```python
from build123d import *

# Parameters (mm, degrees)
SKETCH1_W           = 200
SKETCH1_H           = 200
BOSS_EXTRUDE1_DEPTH = 10
SKETCH2_R           = 5
SKETCH2_R_2         = 2.15
CUT_EXTRUDE1_DEPTH  = 142.774468788
SKETCH3_W           = 20
SKETCH3_H           = 5
SKETCH4_R           = 12.5
SKETCH4_R_2         = 5
SKETCH4_R_3         = 7.5
SKETCH4_R_4         = 2.15
CUT_EXTRUDE2_DEPTH  = 5
BOSS_EXTRUDE3_DEPTH = 1


with BuildPart() as part:
    # Sketch1 → Boss-Extrude1 (new body)
    with BuildSketch(Plane.XY):
        Rectangle(SKETCH1_W, SKETCH1_H)
    extrude(amount=BOSS_EXTRUDE1_DEPTH)

    # Sketch2 → Cut-Extrude1 (cut, through all)
    with BuildSketch(Plane.XY.offset(10)):
        with Locations((-40, 30)):
            Circle(SKETCH2_R)
        with Locations((40, 30)):
            Circle(SKETCH2_R)
        with Locations((40, -30)):
            Circle(SKETCH2_R)
        with Locations((-40, -30)):
            Circle(SKETCH2_R)
        with Locations((-30, 40)):
            Circle(SKETCH2_R)
        with Locations((30, 40)):
            Circle(SKETCH2_R)
        with Locations((30, -40)):
            Circle(SKETCH2_R)
        with Locations((-30, -40)):
            Circle(SKETCH2_R)
        with Locations((-56.6, 90.4)):
            Circle(SKETCH2_R_2)
        with Locations((-90.4, 56.6)):
            Circle(SKETCH2_R_2)
        with Locations((-90.4, -56.6)):
            Circle(SKETCH2_R_2)
        with Locations((-56.6, -90.4)):
            Circle(SKETCH2_R_2)
        with Locations((56.6, -90.4)):
            Circle(SKETCH2_R_2)
        with Locations((90.4, -56.6)):
            Circle(SKETCH2_R_2)
        with Locations((90.4, 56.6)):
            Circle(SKETCH2_R_2)
        with Locations((56.6, 90.4)):
            Circle(SKETCH2_R_2)
    extrude(amount=-CUT_EXTRUDE1_DEPTH, mode=Mode.SUBTRACT)

    # Sketch3 → Cut-Revolve1 (revolve, cut)
    with BuildSketch(Plane(origin=(0, 0, 0), x_dir=(1, 0, 0), z_dir=(0, 1, 0))):
        with Locations((0, -4.492265688)):
            Rectangle(SKETCH3_W, SKETCH3_H)
    revolve(axis=Axis((0, 0, 354.492265688), (1, 0, 0)), mode=Mode.SUBTRACT)

    # Sketch4 → Cut-Extrude2 (cut)
    # profile 1 of 30: a face of its own
    with BuildSketch(Plane.XY.offset(10)):
        with Locations((40, 30)):
            Circle(SKETCH4_R)
    # profile 2 of 30: a face of its own
    with BuildSketch(Plane.XY.offset(10)):
        with Locations((30, 40)):
            Circle(SKETCH4_R)
        with Locations((30, 40)):
            Circle(SKETCH4_R_2, mode=Mode.SUBTRACT)
    # profile 3 of 30: a face of its own
    with BuildSketch(Plane.XY.offset(10)):
        with Locations((30, 40)):
            Circle(SKETCH4_R)
        with Locations((30, 40)):
            Circle(SKETCH4_R_2, mode=Mode.SUBTRACT)
    # profile 4 of 30: a face of its own
    with BuildSketch(Plane.XY.offset(10)):
        with Locations((40, 30)):
            Circle(SKETCH4_R)
        with Locations((40, 30)):
            Circle(SKETCH4_R_2, mode=Mode.SUBTRACT)
    # profile 5 of 30: a face of its own
    with BuildSketch(Plane.XY.offset(10)):
        with Locations((30, 40)):
            Circle(SKETCH4_R)
    # profile 6 of 30: a face of its own
    with BuildSketch(Plane.XY.offset(10)):
        with Locations((40, 30)):
            Circle(SKETCH4_R)
        with Locations((40, 30)):
            Circle(SKETCH4_R_2, mode=Mode.SUBTRACT)
    # profile 7 of 30: a face of its own
    with BuildSketch(Plane.XY.offset(10)):
        with Locations((30, -40)):
            Circle(SKETCH4_R)
    # profile 8 of 30: a face of its own
    with BuildSketch(Plane.XY.offset(10)):
        with Locations((40, -30)):
            Circle(SKETCH4_R)
        with Locations((40, -30)):
            Circle(SKETCH4_R_2, mode=Mode.SUBTRACT)
    # profile 9 of 30: a face of its own
    with BuildSketch(Plane.XY.offset(10)):
        with Locations((30, -40)):
            Circle(SKETCH4_R)
        with Locations((30, -40)):
            Circle(SKETCH4_R_2, mode=Mode.SUBTRACT)
    # profile 10 of 30: a face of its own
    with BuildSketch(Plane.XY.offset(10)):
        with Locations((40, -30)):
            Circle(SKETCH4_R)
        with Locations((40, -30)):
            Circle(SKETCH4_R_2, mode=Mode.SUBTRACT)
    # profile 11 of 30: a face of its own
    with BuildSketch(Plane.XY.offset(10)):
        with Locations((40, -30)):
            Circle(SKETCH4_R)
    # profile 12 of 30: a face of its own
    with BuildSketch(Plane.XY.offset(10)):
        with Locations((30, -40)):
            Circle(SKETCH4_R)
        with Locations((30, -40)):
            Circle(SKETCH4_R_2, mode=Mode.SUBTRACT)
    # profile 13 of 30: a face of its own
    with BuildSketch(Plane.XY.offset(10)):
        with Locations((-30, -40)):
            Circle(SKETCH4_R)
    # profile 14 of 30: a face of its own
    with BuildSketch(Plane.XY.offset(10)):
        with Locations((-40, -30)):
            Circle(SKETCH4_R)
        with Locations((-40, -30)):
            Circle(SKETCH4_R_2, mode=Mode.SUBTRACT)
    # profile 15 of 30: a face of its own
    with BuildSketch(Plane.XY.offset(10)):
        with Locations((-30, -40)):
            Circle(SKETCH4_R)
        with Locations((-30, -40)):
            Circle(SKETCH4_R_2, mode=Mode.SUBTRACT)
    # profile 16 of 30: a face of its own
    with BuildSketch(Plane.XY.offset(10)):
        with Locations((-40, -30)):
            Circle(SKETCH4_R)
        with Locations((-40, -30)):
            Circle(SKETCH4_R_2, mode=Mode.SUBTRACT)
    # profile 17 of 30: a face of its own
    with BuildSketch(Plane.XY.offset(10)):
        with Locations((-40, 30)):
            Circle(SKETCH4_R)
    # profile 18 of 30: a face of its own
    with BuildSketch(Plane.XY.offset(10)):
        with Locations((-30, 40)):
            Circle(SKETCH4_R)
        with Locations((-30, 40)):
            Circle(SKETCH4_R_2, mode=Mode.SUBTRACT)
    # profile 19 of 30: a face of its own
    with BuildSketch(Plane.XY.offset(10)):
        with Locations((-40, 30)):
            Circle(SKETCH4_R)
        with Locations((-40, 30)):
            Circle(SKETCH4_R_2, mode=Mode.SUBTRACT)
    # profile 20 of 30: a face of its own
    with BuildSketch(Plane.XY.offset(10)):
        with Locations((-30, 40)):
            Circle(SKETCH4_R)
        with Locations((-30, 40)):
            Circle(SKETCH4_R_2, mode=Mode.SUBTRACT)
    # profile 21 of 30: a face of its own
    with BuildSketch(Plane.XY.offset(10)):
        with Locations((-30, 40)):
            Circle(SKETCH4_R)
    # profile 22 of 30: a face of its own
    with BuildSketch(Plane.XY.offset(10)):
        with Locations((-40, 30)):
            Circle(SKETCH4_R)
        with Locations((-40, 30)):
            Circle(SKETCH4_R_2, mode=Mode.SUBTRACT)
    # profile 23 of 30: a face of its own
    with BuildSketch(Plane.XY.offset(10)):
        with Locations((-56.6, 90.4)):
            Circle(SKETCH4_R_3)
        with Locations((-56.6, 90.4)):
            Circle(SKETCH4_R_4, mode=Mode.SUBTRACT)
    # profile 24 of 30: a face of its own
    with BuildSketch(Plane.XY.offset(10)):
        with Locations((-90.4, 56.6)):
            Circle(SKETCH4_R_3)
        with Locations((-90.4, 56.6)):
            Circle(SKETCH4_R_4, mode=Mode.SUBTRACT)
    # profile 25 of 30: a face of its own
    with BuildSketch(Plane.XY.offset(10)):
        with Locations((56.6, -90.4)):
            Circle(SKETCH4_R_3)
        with Locations((56.6, -90.4)):
            Circle(SKETCH4_R_4, mode=Mode.SUBTRACT)
    # profile 26 of 30: a face of its own
    with BuildSketch(Plane.XY.offset(10)):
        with Locations((90.4, -56.6)):
            Circle(SKETCH4_R_3)
        with Locations((90.4, -56.6)):
            Circle(SKETCH4_R_4, mode=Mode.SUBTRACT)
    # profile 27 of 30: a face of its own
    with BuildSketch(Plane.XY.offset(10)):
        with Locations((90.4, 56.6)):
            Circle(SKETCH4_R_3)
        with Locations((90.4, 56.6)):
            Circle(SKETCH4_R_4, mode=Mode.SUBTRACT)
    # profile 28 of 30: a face of its own
    with BuildSketch(Plane.XY.offset(10)):
        with Locations((56.6, 90.4)):
            Circle(SKETCH4_R_3)
        with Locations((56.6, 90.4)):
            Circle(SKETCH4_R_4, mode=Mode.SUBTRACT)
    # profile 29 of 30: a face of its own
    with BuildSketch(Plane.XY.offset(10)):
        with Locations((-90.4, -56.6)):
            Circle(SKETCH4_R_3)
    # profile 30 of 30: a face of its own
    with BuildSketch(Plane.XY.offset(10)):
        with Locations((-56.6, -90.4)):
            Circle(SKETCH4_R_3)
    extrude(amount=-CUT_EXTRUDE2_DEPTH, mode=Mode.SUBTRACT)

    # Sketch6 → Boss-Extrude3 (add)
    with BuildSketch(Plane.XY.offset(10)):
        Polygon((10, -45.621583501), (0, -45.621583501), (10, -60.912010155), align=None)
        Polygon((-10, -45.621583501), (0, -45.621583501), (10, -45.621583501), (10, -37.997610078), (-10, -37.997610078), align=None)
        Polygon((-10, -60.912010155), (0, -45.621583501), (-10, -45.621583501), align=None)
    extrude(amount=-BOSS_EXTRUDE3_DEPTH)


solid = part.part
```
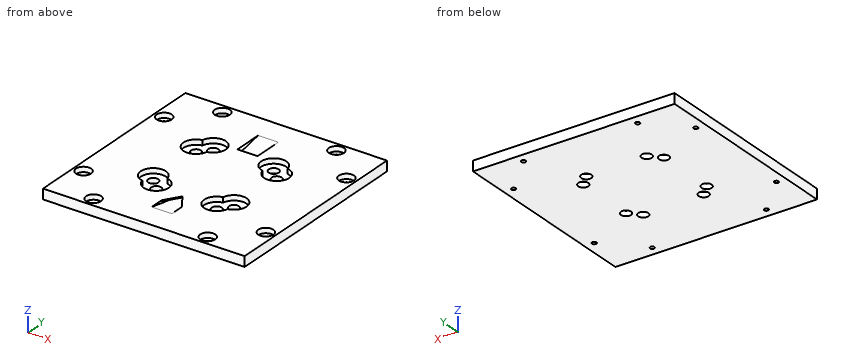
The model under review builds one solid part; all positions refer to its coordinate system, in mm. Coordinates: 2 decimals unless noted, no trailing zeros. Write each loop counter-clockwise with the first axis right and the second up, starting at its lowest first coordinate (ties: lowest second). Pieces come first, ordered by that corner, then holes. Notation, with made-up numbers: (-12.75, -5) - (33.25, -5) arc R21 cw to (33.25, 15) - close; hole circle Ø1 at (-21.75, 19). An arc over 180 degrees is marked (long way). Answer in a Markdown table with one row per item. Add a question column.
Q1. Consider section C-C on y = -15. Give the boundary of the cut face in (x, z), then the cut area to 3 significant figures.
Q2. Clearance check with a flat-ended pin moving along its axis: pin 1 (20 mm diameter, centred on x = 30, y = -40, fed in from +Z). State where the tip first meets the part, or that it passes through.
Q3. Consider section D-D on y = 6. Give the boundary of the cut face in (x, z), then the cut area to 3 significant figures.
Q4. Consider section B-B on x = 30. Give the boundary of the cut face in (y, z).
Q5. To check wall thickness, follow line 1 along Y through (x, z) = (-40, 2.5); line 2 along Y through (x, z) = (-56.6, 2.4); line 3 along X through (y, z) = (90.5, 2.5). State the ranges of each line that lie inside material, in increasing order. Write a range as from..to.
Q6. Consider section A-A on y = 32.5. Give the boundary of the cut face in (x, z).
Answers below:
| question | item | result |
|---|---|---|
| 1 | outline | (-100, 0) - (100, 0) - (100, 10) - (-100, 10) - close; hole (-10, 2.31) - (10, 2.31) - (10, 7.32) - (-10, 7.32) - close |
| 1 | area | 1,900 mm² |
| 2 | pin 1 | z = 5 |
| 3 | outline | (-100, 0) - (100, 0) - (100, 10) - (-100, 10) - close; hole (-10, 2.04) - (10, 2.04) - (10, 7.04) - (-10, 7.04) - close |
| 3 | area | 1,900 mm² |
| 4 | outline | (-100, 0) - (-45, 0) - (-45, 5) - (-52.5, 5) - (-52.5, 10) - (-100, 10) - close; (-35, 0) - (35, 0) - (35, 5) - (22.5, 5) - (22.5, 10) - (-22.5, 10) - (-22.5, 5) - (-35, 5) - close; (45, 0) - (100, 0) - (100, 10) - (52.5, 10) - (52.5, 5) - (45, 5) - close |
| 5 | line 1 | -100..-35, -25..25, 35..100 |
| 5 | line 2 | -100..-92.55, -88.25..88.25, 92.55..100 |
| 5 | line 3 | -100..-58.75, -54.45..54.45, 58.75..100 |
| 6 | outline | (-100, 0) - (-44.33, 0) - (-44.33, 5) - (-52.25, 5) - (-52.25, 10) - (-100, 10) - close; (-35.67, 0) - (35.67, 0) - (35.67, 5) - (20, 5) - (20, 10) - (-20, 10) - (-20, 5) - (-35.67, 5) - close; (44.33, 0) - (100, 0) - (100, 10) - (52.25, 10) - (52.25, 5) - (44.33, 5) - close; hole (-10, 3.49) - (10, 3.49) - (10, 8.52) - (-10, 8.52) - close |
